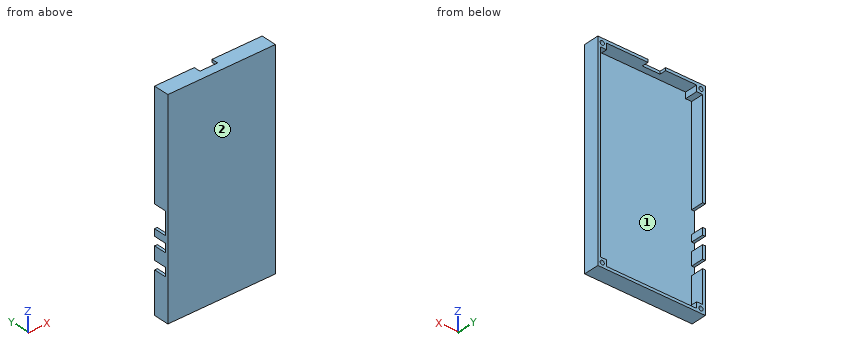
Autodesk Inventor part; units mm, degrees
ref_plane "YZ Plane" through (0, 0, 0) normal (1, 0, 0) x (0, 1, 0)
ref_plane "XZ Plane" through (0, 0, 0) normal (0, 1, 0) x (-1, 0, 0)
ref_plane "XY Plane" through (0, 0, 0) normal (0, 0, 1) x (1, 0, 0)
sketch "Sketch1" plane through (0, 0, 0) normal (0, 1, 0) x (-1, 0, 0)
  line L0 (0, 0) -> (62.23, 0)
  line L1 (62.23, 0) -> (62.23, -120.65)
  line L2 (62.23, -120.65) -> (0, -120.65)
  line L3 (0, -120.65) -> (0, 0)
  dimension "d0" = 62.23
  dimension "d1" = 120.65
extrude "Extrusion1" add sketch "Sketch1" along normal blind 1.5
sketch "Sketch2" plane through (0, 1.5, 0) normal (0, 1, 0) x (1, 0, 0)
  line L0 (-60.6425, 1.5875) -> (-1.5875, 1.5875)
  line L1 (-1.5875, 1.5875) -> (-1.5875, 119.0625)
  line L2 (-1.5875, 119.0625) -> (-60.6425, 119.0625)
  line L3 (-60.6425, 119.0625) -> (-60.6425, 1.5875)
  line L4 (-62.23, 0) -> (0, 0)
  line L5 (0, 0) -> (0, 120.65)
  line L6 (-62.23, 120.65) -> (-62.23, 0)
  line L7 (0, 120.65) -> (-62.23, 120.65)
  line L8 (0, 0) -> (-5.08, 0)
  line L9 (-5.08, 0) -> (-5.08, 5.08)
  line L10 (-5.08, 5.08) -> (0, 5.08)
  line L11 (0, 5.08) -> (0, 0)
  line L12 (-62.23, 0) -> (-57.15, 0)
  line L13 (-57.15, 0) -> (-57.15, 5.08)
  line L14 (-57.15, 5.08) -> (-62.23, 5.08)
  line L15 (-62.23, 5.08) -> (-62.23, 0)
  line L16 (0, 120.65) -> (-5.08, 120.65)
  line L17 (-5.08, 120.65) -> (-5.08, 115.57)
  line L18 (-5.08, 115.57) -> (0, 115.57)
  line L19 (0, 115.57) -> (0, 120.65)
  line L20 (-62.23, 120.65) -> (-57.15, 120.65)
  line L21 (-57.15, 120.65) -> (-57.15, 115.57)
  line L22 (-57.15, 115.57) -> (-62.23, 115.57)
  line L23 (-62.23, 115.57) -> (-62.23, 120.65)
  point P0 (0, 115.57)
  point P1 (-1.5875, 115.57)
  point P2 (-1.5875, 5.08)
  point P3 (-5.08, 1.5875)
  point P4 (-57.15, 1.5875)
  point P5 (-60.6425, 5.08)
  point P6 (-5.08, 119.0625)
  point P7 (-60.6425, 115.57)
  point P8 (-57.15, 119.0625)
  dimension "d4" = 1.5875
  dimension "d5" = 1.5875
  dimension "d6" = 1.5875
  dimension "d7" = 1.5875
  dimension "d8" = 5.08
  dimension "d9" = 5.08
  dimension "d10" = 5.08
  dimension "d11" = 5.08
  dimension "d12" = 5.08
  dimension "d13" = 5.08
  dimension "d14" = 5.08
  dimension "d15" = 5.08
extrude "Extrusion3" add sketch "Sketch2" along normal blind 7.5 contours L3 L14 L13 L0 | L0 L13 L4 L6 L14 L3 | L0 L9 L4 L13 | L14 L6 L22 L3 | L9 L10 L1 L0 | L0 L1 L10 L5 L4 L9 | L22 L6 L7 L21 L2 L3 | L3 L2 L21 L22 | L1 L18 L5 L10 | L21 L7 L17 L2 | L18 L17 L2 L1 | L1 L2 L17 L7 L5 L18
sketch "Sketch3" plane through (0, 9, 0) normal (0, 1, 0) x (1, 0, 0)
  line L0 (-62.23, 0) -> (0, 0)
  line L1 (-39.23, 0) -> (-29, 0)
  line L2 (-29, 0) -> (-29, 1.5875)
  line L3 (-29, 1.5875) -> (-39.23, 1.5875)
  line L4 (-39.23, 1.5875) -> (-39.23, 0)
  line L5 (0, 0) -> (0, 120.65)
  line L6 (-62.23, 120.65) -> (-62.23, 0)
  line L7 (0, 120.65) -> (-62.23, 120.65)
  line L8 (-60.6425, 115.57) -> (-60.6425, 5.08)
  line L9 (-62.23, 60.325) -> (-60.6425, 60.325)
  line L10 (-60.6425, 60.325) -> (-60.6425, 98.425)
  line L11 (-60.6425, 98.425) -> (-62.23, 98.425)
  line L12 (-62.23, 98.425) -> (-62.23, 60.325)
  point P0 (-59.69, 2.54)
  point P1 (-59.69, 118.11)
  point P2 (-2.54, 118.11)
  point P3 (-2.54, 2.54)
  dimension "d20" = 29
  dimension "d21" = 23
  dimension "d22" = 2.54
  dimension "d23" = 2.54
  dimension "d24" = 2.54
  dimension "d25" = 2.54
  dimension "d26" = 2.54
  dimension "d27" = 2.54
  dimension "d28" = 2.54
  dimension "d29" = 2.54
  dimension "d47" = 60.325
  dimension "d48" = 22.225
extrude "Extrusion4" cut sketch "Sketch3" against normal blind 3.81 contours L4 L3 L2 L0
sketch "Sketch4" plane through (0, 9, 0) normal (0, 1, 0) x (1, 0, 0)
  line L0 (-29, 0) -> (0, 0)
  line L1 (0, 0) -> (0, 120.65)
  line L2 (-62.23, 0) -> (-39.23, 0)
  line L3 (-62.23, 120.65) -> (-62.23, 0)
  line L4 (0, 120.65) -> (-62.23, 120.65)
  point P0 (-2.54, 2.54)
  point P1 (-2.54, 118.11)
  point P2 (-59.69, 118.11)
  point P3 (-59.69, 2.54)
  dimension "d39" = 2.54
  dimension "d40" = 2.54
  dimension "d41" = 2.54
  dimension "d42" = 2.54
  dimension "d43" = 2.54
  dimension "d44" = 2.54
  dimension "d45" = 2.54
  dimension "d46" = 2.54
hole "Hole1" at (-2.54, 9, -2.54) at (-2.54, 9, -118.11) at (-59.69, 9, -118.11) at (-59.69, 9, -2.54) direction (0, -1, 0) diameter 2.4384 depth 5.08
sketch "Sketch5" plane through (0, 9, 0) normal (0, 1, 0) x (1, 0, 0)
  line L0 (-62.23, 91.65) -> (-60.6425, 91.65)
  line L1 (-60.6425, 5.08) -> (-60.6425, 115.57)
  line L2 (-62.23, 120.65) -> (-62.23, 0)
  line L3 (-62.23, 79) -> (-60.6425, 79)
  line L4 (-62.23, 84) -> (-60.6425, 84)
  line L5 (-62.23, 75) -> (-60.6425, 75)
  line L6 (-62.23, 62) -> (-60.6425, 62)
  line L7 (-62.23, 0) -> (-39.23, 0)
  line L8 (0, 120.65) -> (-62.23, 120.65)
  line L9 (-62.23, 96.65) -> (-60.6425, 96.65)
  point P0 (0, 0)
  dimension "d49" = 62
  dimension "d50" = 75
  dimension "d51" = 79
  dimension "d52" = 5
  dimension "d53" = 29
  dimension "d54" = 5
extrude "Extrusion5" cut sketch "Sketch5" against normal up to surface (7.5 mm away) contours L2 L9 L1 L0 | L4 L1 L3 L2 | L5 L1 L6 L2
equation "\"d4\" = d5"
equation "\"d6\" = d5"
equation "\"d7\" = d5"
equation "\"d10\" = d8"
equation "\"d11\" = d10"
equation "\"d12\" = d8"
equation "\"d13\" = d8"
equation "\"d14\" = d8"
equation "\"d15\" = d8"
properties part number "cover_bottom"
The listing builds one solid part. Answer for the finished solid, in the listing's coordinates (mm). Face numbers are marked on the shaded views. Round coordinates to 2 decimals unless told otherwise and drop trailing zeros. Loops run counter-clockwise (first coordinate to the right, second up) from the corner with the lowest first, then second, coordinate; pieces in that order, holes last.
1) For a pull along Z with two mould halves and no side action, classify the marked faces 1 and 2 as released by +Z, released by -Z, zero draft, split by the parting line, or undercut.
Outcome:
face 1: undercut
face 2: zero draft
2) A cutting plane is placed at A-A on y = 2.75. Determine the outline of the cut face in (x, z), plus the area to 3 significant figures.
Outcome:
outline: (-62.23, -120.65) - (0, -120.65) - (0, 0) - (-62.23, 0) - (-62.23, -62) - (-60.64, -62) - (-60.64, -5.08) - (-57.15, -5.08) - (-57.15, -1.59) - (-5.08, -1.59) - (-5.08, -5.08) - (-1.59, -5.08) - (-1.59, -115.57) - (-5.08, -115.57) - (-5.08, -119.06) - (-57.15, -119.06) - (-57.15, -115.57) - (-60.64, -115.57) - (-60.64, -96.65) - (-62.23, -96.65) - close; (-62.23, -91.65) - (-60.64, -91.65) - (-60.64, -84) - (-62.23, -84) - close; (-62.23, -79) - (-60.64, -79) - (-60.64, -75) - (-62.23, -75) - close
area: 583 mm2
3) A cutting plane is placed at B-B on z = -108. Determine the outline of the cut face in (x, y), plus the area to 3 significant figures.
Outcome:
outline: (-62.23, 0) - (0, 0) - (0, 9) - (-1.59, 9) - (-1.59, 1.5) - (-60.64, 1.5) - (-60.64, 9) - (-62.23, 9) - close
area: 117 mm2
4) Consider line 1 (Z direction, x = -59.69, y = 5.6); line 2 (X direction, y = 7.1, z = -2.54); line 3 (X direction, y = 4.5, z = -56). Determine where each line is inside the solid, lowest interval first.
Outcome:
line 1: z = -120.65 to -119.33, -116.89 to -115.57, -5.08 to -3.76, -1.32 to 0
line 2: x = -62.23 to -60.91, -58.47 to -57.15, -5.08 to -3.76, -1.32 to 0
line 3: x = -62.23 to -60.64, -1.59 to 0
5) Given P1, Ø0.7, axis at x = -60, z = -2.5, coming from the +Y side; P2, Ø8, axis at x = -8, z = -30.5, coming from the +Y side; P3, Ø0.8, axis at x = -34.5, z = -0.5, coming from the +Y side, each flat-ended and moving along its own axis, determine where each tip first touches the part or whether it passes through.
Outcome:
P1: stops at y = 3.92
P2: stops at y = 1.5
P3: stops at y = 5.19
6) A cutting plane is placed at C-C on x = -37. Determine the outline of the cut face in (y, z), plus the area to 3 significant figures.
Outcome:
outline: (0, -120.65) - (9, -120.65) - (9, -119.06) - (1.5, -119.06) - (1.5, -1.59) - (5.19, -1.59) - (5.19, 0) - (0, 0) - close
area: 199 mm2
